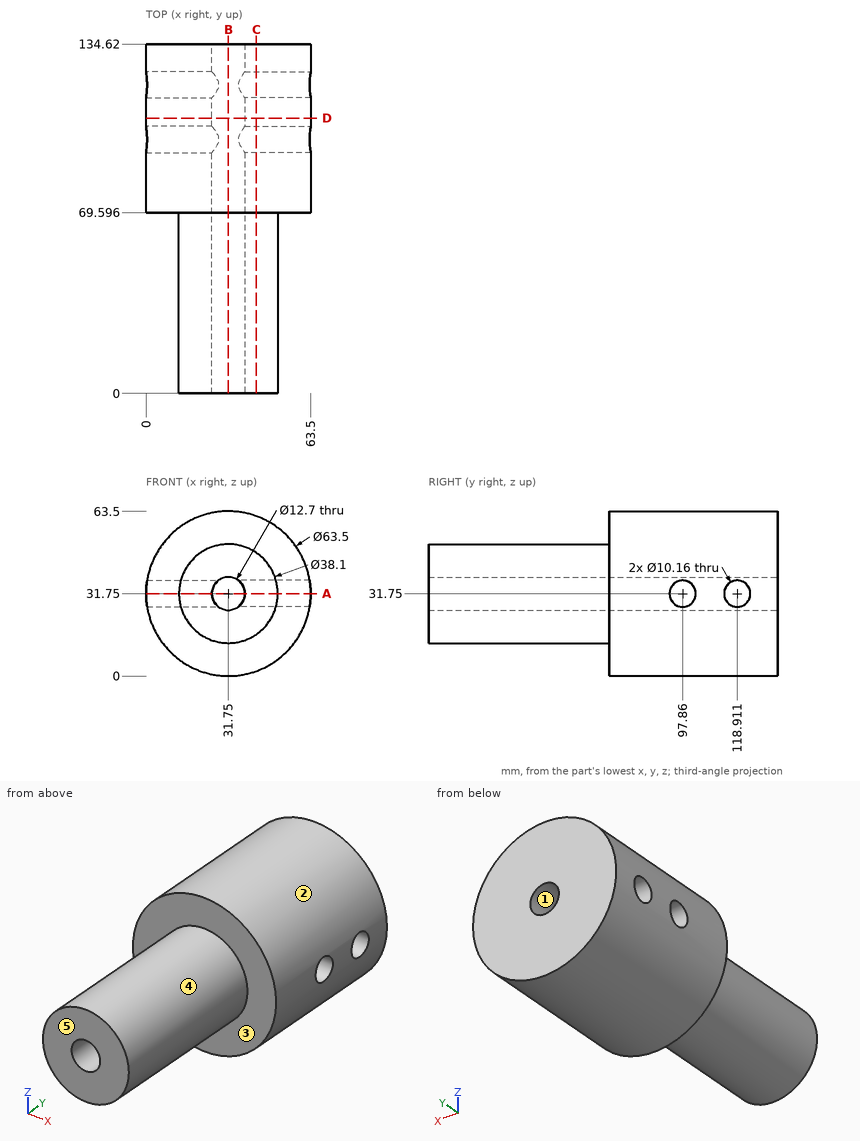
Could you check a few things on this drawing? It's one solid part, dimensions in mm from its lowest x, y, z. A direction names the side the tool comes from. Give positions to 0.01 mm unless a question says otherwise; leave off trailing zeros. Loops run counter-clockwise (first coordinate to the right, second up) from the corner with the lowest first, then second, coordinate; pieces in that order, holes last. Notation, with made-up numbers: M 68.5,10.5 L 104.5,10.5 A31 cw 104.5,40.5 Z; hole C 62,79 d3. An arc over 180 degrees is marked long. Return JSON: item names as keys, results as strings.
Item 1: Imagine slicing it at D-D on y = 106. List the corners of the cut face in (x, z) for me.
A:
{"outline": "C 31.75,31.75 d63.5; hole C 31.75,31.75 d12.7"}
Item 2: Please list where these lines run through material, in increasing order: line 1 (Y direction, x = 52, z = 31) (1 decimal); line 2 (Y direction, x = 50, z = 31) (1 decimal); line 3 (Y direction, x = 60, z = 45).
A:
{"line 1": "y = 69.6 to 92.8, 102.9 to 113.9, 123.9 to 134.6", "line 2": "y = 0 to 92.8, 102.9 to 113.9, 123.9 to 134.6", "line 3": "y = 69.6 to 134.62"}
Item 3: Imagine slicing it at C-C on x = 42.5. State how many separate pieces and enclosed holes the cut face has, then the cut area to 3 significant figures.
A:
{"separate pieces": "1", "enclosed holes": "2", "area": "5,910 mm^2"}
Item 4: On a 3-axis mill with a long thin cutter (end or side, diameter ignored), from which of +Z, -Z, +X, -X, +Y, -Y can I reach the whole of each face in a straight line? I mean the marked faces 4 and 5. Say none if no direction works.
A:
{"face 4": "-Y", "face 5": "+Z, -Z, +X, -X, -Y"}
Item 5: Thinking about a two-plate mould opening in Z: for the marked faces 1, 2 and 3, which applies, released by +Z, released by -Z, zero draft, split by the parting line, or undercut?
A:
{"face 1": "undercut", "face 2": "split by the parting line", "face 3": "zero draft"}
Item 6: I'm going to push flat-ended pins straight in: pin 1 Ø8 at (y, z) = (70.5, 14.5) entering from -X; pin 2 Ø6 at (x, y) = (8.5, 70) entering from +Z (1 decimal); pin 3 Ø12 at (x, y) = (26.5, 59.5) entering from -Z. Where does each tip first touch, or does it pass through?
A:
{"pin 1": "stops at x = 2.9", "pin 2": "stops at z = 56.2", "pin 3": "stops at z = 12.7"}
Item 7: Imagine slicing it at A-A on z = 31.75. List the corners of the cut face in (x, y) for me, then the cut area to 3 significant figures.
A:
{"outline": "M 0,69.6 L 12.7,69.6 L 12.7,0 L 25.4,0 L 25.4,92.78 L 0,92.78 Z; M 0,102.94 L 25.4,102.94 L 25.4,113.83 L 0,113.83 Z; M 0,123.99 L 25.4,123.99 L 25.4,134.62 L 0,134.62 Z; M 38.1,0 L 50.8,0 L 50.8,69.6 L 63.5,69.6 L 63.5,92.78 L 38.1,92.78 Z; M 38.1,102.94 L 63.5,102.94 L 63.5,113.83 L 38.1,113.83 Z; M 38.1,123.99 L 63.5,123.99 L 63.5,134.62 L 38.1,134.62 Z", "area": "4,040 mm^2"}
Item 8: Imagine slicing it at B-B on x = 31.75. List the corners of the cut face in (y, z) for me.
A:
{"outline": "M 0,12.7 L 69.6,12.7 L 69.6,0 L 134.62,0 L 134.62,25.4 L 0,25.4 Z; M 0,38.1 L 134.62,38.1 L 134.62,63.5 L 69.6,63.5 L 69.6,50.8 L 0,50.8 Z"}
